Design review of the part built by this model. Coordinates are the model's own, in mm. A direction names the side the tool comes from. Round coordinates to 2 decimals unless told otherwise and drop trailing zeros. Loops run counter-clockwise (first coordinate to the right, second up) from the corner with the lowest first, then second, coordinate; pieces in that order, holes last. Notation, with made-up numbers: (82.25, -7) - (105.25, -7) arc R7 cw to (105.25, 1) - close; hole circle Ø11 at (-2.5, -28). An arc over 180 degrees is marked (long way). Use one line per item in the form item = value. Start each with the question number.
(1) Machinability: for faces 4 (the flat face through (9.5, -17.5, 61.799)), 5 (the cylindrical face through (-14.536, 4.578, 11.683)), 6 (the cylindrical face through (-18.17, 5.72, 50.13)), which of the approach directions +Z, -Z, +X, -X, +Y, -Y give a long, thin tool a straight path to every point of the face, cutting with its end or side? Answer none if there is none.
(2) We need section B-B, the plane z = 40.5. Write out the cut boundary in (x, y).
(3) For pin 1 (12 mm diameter, centred on x = 8.5, y = 2, fed in from +Z); pin 2 (5 mm diameter, centred on x = 7, z = 21.5, fed in from -Y); pin 3 (1.5 mm diameter, centred on y = -9, z = 23, fed in from +X); pin 4 (6 mm diameter, centred on x = 6.5, y = 12, fed in from -Z), all flat-tipped, find the tip position at first contact; note any pin that passes through.
(4) The part is to be moulded in two halves that separate along Y. For faces 1 (the cylindrical face through (15.913, 14.592, 49.783)), 2 (the conical face through (-13.202, 4.158, 28.058)), 3 (the flat face through (0.1, -13.5, 0)), say which applies: released by +Y, released by -Y, zero draft, split by the parting line, or undercut.
(5) We need section A-A, the plane z = 17. Write out the cut boundary in (x, y), then the cut area to 3 significant figures.
(6) Wall thickness on probe 1 along X at (y, z) = (0, 49); probe 2 along X at (y, z) = (0, 7): over which ranges is each line inside the solid? List them lowest first. Write a range as [from, to].
from build123d import *

# Parameters (mm, degrees)
F2_R    = 6.35
F3_SIZE = 0.635


with BuildPart() as f1:
    # F0 (on Front) → F1 (revolve)
    with BuildSketch(Plane.XZ):
        Polygon((-19.05, 61.798523), (-21.59, 61.798523), (-21.59, 36.398523), (-15.24, 25.4), (-15.24, 0), (-12.7, 0), (-12.7, 26.080591), (-19.05, 37.079114), align=None)
    revolve(axis=Axis((0, 0, 30.899261), (0, 0, -1)))

    # F2
    f2_edges = [f1.edges().sort_by_distance(p)[0] for p in [
        (21.59, 0, 36.398523),
        (15.24, 0, 25.4),
        (19.05, 0, 37.079114),
        (12.7, 0, 26.080591),
    ]]
    fillet(f2_edges, radius=F2_R)

    # F3
    f3_edges = [f1.edges().sort_by_distance(p)[0] for p in [
        (12.7, 0, 0),
        (19.05, 0, 61.798523),
    ]]
    chamfer(f3_edges, length=F3_SIZE)


solid = f1.part
Data:
q1.face_4 = +Z, +X, -X, +Y, -Y
q1.face_5 = -Z
q1.face_6 = +Z
q2.outline = circle Ø43.18 at (0, 0); hole circle Ø38.1 at (0, 0)
q3.pin_1 = 29.6
q3.pin_2 = -14.56
q3.pin_3 = 12.81
q3.pin_4 = 0
q4.face_1 = split by the parting line
q4.face_2 = undercut
q4.face_3 = zero draft
q5.outline = circle Ø30.48 at (0, 0); hole circle Ø25.4 at (0, 0)
q5.area = 223 mm^2
q6.probe_1 = [-21.59, -19.05], [19.05, 21.59]
q6.probe_2 = [-15.24, -12.7], [12.7, 15.24]
